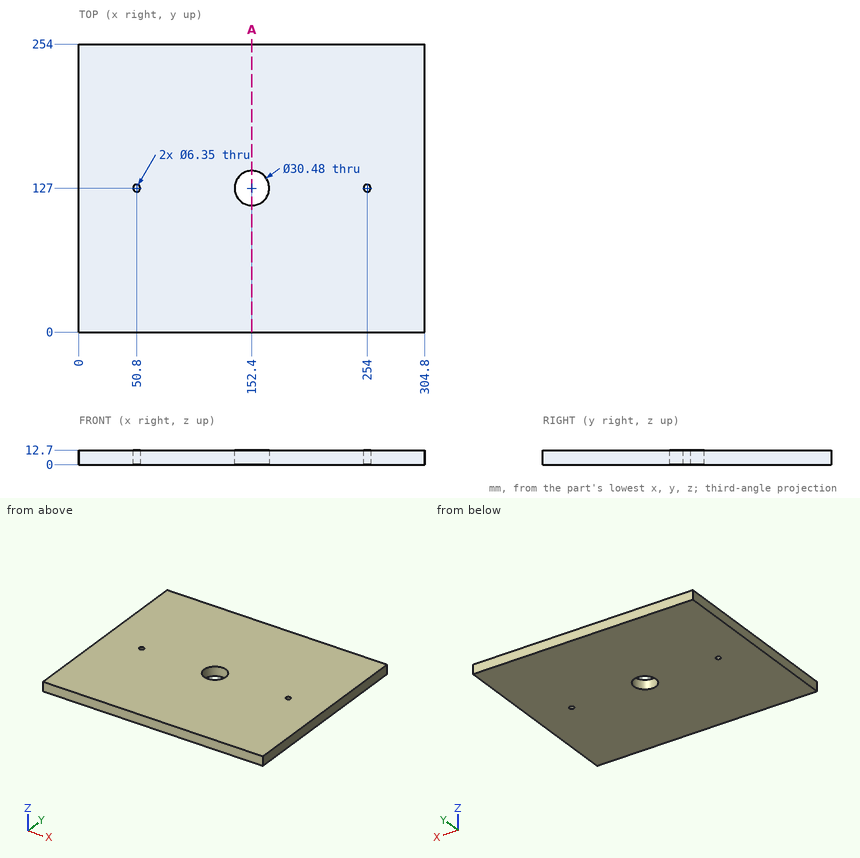
Geometry: see drawing. Coordinates: mm, zero at the bounding-box minimum. Round coordinates to 2 decimals unless told otherwise and drop trailing zeros. Loops run counter-clockwise (first coordinate to the right, second up) from the corner with the lowest first, then second, coordinate; pieces in that order, holes last. Notation, with made-up numbers: (28.5, -10.75) - (41.5, -10.75) arc R24 ccw to (41.5, 0.25) - close; hole circle Ø6 at (-3.5, 74). An arc over 180 degrees is marked (long way). Write item = value, one per line. Start each with the question number.
(1) Ray query, line 1 along Y through (x, z) = (50.8, 9) (3 decimals); line 2 along Y through (x, z) = (142, 6.75). Return the intervals inside material, ascending. Write a range as from..to.
(2) Pin query (flat end, axial travel): pin 1 (1.5 mm diameter, centred on x = 268.5, y = 181, fed in from -Z). Return the tip coordinate at first contact, or that it passes through.
(3) Section query A-A, the plane x = 152.4. Output: boundary loops of the cut face in (y, z), plus the area to 3 significant figures.
Conclusion:
q1.line_1 = 0..123.825, 130.175..254
q1.line_2 = 0..115.86, 138.14..254
q2.pin_1 = 0
q3.outline = (0, 0) - (111.76, 0) - (111.76, 12.7) - (0, 12.7) - close; (142.24, 0) - (254, 0) - (254, 12.7) - (142.24, 12.7) - close
q3.area = 2,840 mm2
